CAD build for the part. Positions are in the model's coordinates, mm. Face numbers are marked on the shaded views. A direction names the side the tool comes from. Coordinates: 2 decimals unless noted, no trailing zeros. Loops run counter-clockwise (first coordinate to the right, second up) from the corner with the lowest first, then second, coordinate; pieces in that order, holes last. Notation, with made-up numbers: (64.25, 19) -> (81.25, 19) arc R6 ccw to (81.25, 26) -> close; hole circle Ø3 at (-33.5, -14.5). An arc over 180 degrees is marked (long way). Return JSON: item names as keys, results as strings. Group by question number.
(1) Saw through at C-C on y = 5. Write the cut outline in (x, z) (3 decimals), then the cut area to 3 significant figures.
(2) Flat gauge pins, fed straight in: pin 1 Ø6 at (x, z) = (23, -6) entering from +Y; pin 2 Ø1.7 at (y, z) = (-2, 7.5) entering from +X (3 decimals); pin 3 Ø8 at (y, z) = (20, 3.5) entering from +X (3 decimals); pin 4 Ø1 at (x, y) = (18.5, 64) entering from +Z. Where does each tip first touch, or does it go through?
(3) Saw through at D-D on z = 10.75. Write the cut outline in (x, y) (3 decimals), then the cut area to 3 significant figures.
(4) Mould opens along Y. For the marked faces 3, 4, 5 and 6 say: pulls with the +Y half, pulls with the -Y half, needs draft (parallel to the pull), parting line crosses it, or undercut.
(5) Probe L1, parallel to Y at x = 31.75, z = 0.9; L2, parallel to Y at x = 18.5, z = -0.25; L3, parallel to Z at x = 17, y = 22.5. List the from-to ranges inside material, lowest first.
(6) Saw through at B-B on x = 15. Write the cut outline in (y, z).
(7) Saw through at A-A on x = 31.75. Write the cut outline in (y, z).
(8) Tool access for the marked faces 1 and 2: list every direction of +Z, -Z, +X, -X, +Y, -Y with a clear straight run to the whole face (end or side of a thin tool).
```python
from build123d import *

# Parameters (mm, degrees)
SKETCH1_W           = 33.655
SKETCH1_H           = 92.71
SKETCH1_R           = 0.925
BOSS_EXTRUDE1_DEPTH = 1.6
SKETCH2_W           = 33.655
SKETCH2_H           = 74.776129116
BOSS_EXTRUDE2_DEPTH = 11
SKETCH3_W           = 27
SKETCH3_H           = 20.3
BOSS_EXTRUDE3_DEPTH = 5.7


with BuildPart() as part:
    # Sketch1 → Boss-Extrude1 (new body)
    with BuildSketch(Plane.XY):
        with Locations((16.8275, 46.355)):
            Rectangle(SKETCH1_W, SKETCH1_H)
        with Locations((1.905, 90.805)):
            Circle(SKETCH1_R, mode=Mode.SUBTRACT)
        with Locations((31.75, 90.805)):
            Circle(SKETCH1_R, mode=Mode.SUBTRACT)
        with Locations((1.905, 1.905)):
            Circle(SKETCH1_R, mode=Mode.SUBTRACT)
        with Locations((31.75, 1.905)):
            Circle(SKETCH1_R, mode=Mode.SUBTRACT)
    extrude(amount=BOSS_EXTRUDE1_DEPTH)

    # Sketch2 → Boss-Extrude2 (add)
    with BuildSketch(Plane(origin=(0, 0, 0), x_dir=(-1, 0, 0), z_dir=(0, 0, -1))):
        with Locations((-16.8275, 47.192358669)):
            Rectangle(SKETCH2_W, SKETCH2_H)
    extrude(amount=BOSS_EXTRUDE2_DEPTH)

    # Sketch3 → Boss-Extrude3 (add)
    with BuildSketch(Plane.XZ):
        with Locations((16.825, 5.23)):
            Rectangle(SKETCH3_W, SKETCH3_H)
    extrude(amount=BOSS_EXTRUDE3_DEPTH)


solid = part.part
```
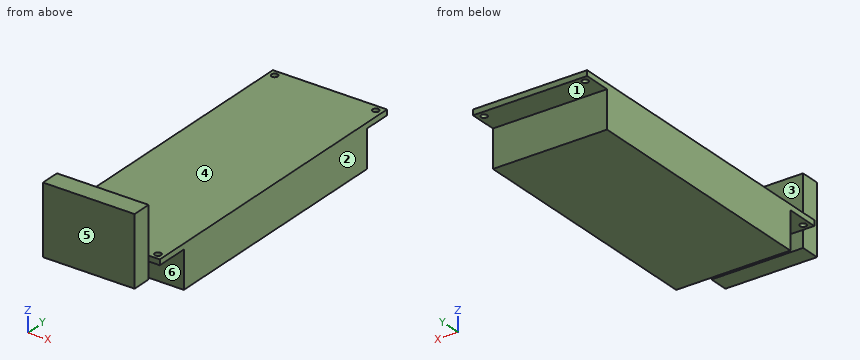
Geometry results:
{
 "1": {"outline": "(0, 0) -> (33.655, 0) -> (33.655, 1.6) -> (0, 1.6) -> close", "area": "53.8 mm²"},
 "2": {"pin 1": "y = 84.58", "pin 2": "x = 30.325", "pin 3": "x = 33.655", "pin 4": "z = 1.6"},
 "3": {"outline": "(3.325, -5.7) -> (30.325, -5.7) -> (30.325, 0) -> (3.325, 0) -> close", "area": "154 mm²"},
 "4": {"face 3": "pulls with the +Y half", "face 4": "needs draft", "face 5": "pulls with the -Y half", "face 6": "undercut"},
 "5": {"L1": "0 to 0.98, 2.83 to 89.88, 91.73 to 92.71", "L2": "-5.7 to 0, 9.8 to 84.58", "L3": "-11 to 1.6"},
 "6": {"outline": "(-5.7, -4.92) -> (0, -4.92) -> (0, 0) -> (9.8, 0) -> (9.8, -11) -> (84.58, -11) -> (84.58, 0) -> (92.71, 0) -> (92.71, 1.6) -> (0, 1.6) -> (0, 15.38) -> (-5.7, 15.38) -> close"},
 "7": {"outline": "(0, 0) -> (0.98, 0) -> (0.98, 1.6) -> (0, 1.6) -> close; (2.83, 0) -> (9.8, 0) -> (9.8, -11) -> (84.58, -11) -> (84.58, 0) -> (89.88, 0) -> (89.88, 1.6) -> (2.83, 1.6) -> close; (91.73, 0) -> (92.71, 0) -> (92.71, 1.6) -> (91.73, 1.6) -> close"},
 "8": {"face 1": "-Z, +X, -X, +Y", "face 2": "+Z, -Z, +X, +Y, -Y"}
}
